CAD build for the part. Positions are in the model's coordinates, mm. A direction names the side the tool comes from. Round coordinates to 2 decimals unless told otherwise and drop trailing zeros. Order: outer loops, then holes, each group sorted by start corner. A loop starts at its lowest first (then second) coordinate and runs counter-clockwise, first axis right, second up. Notation, with made-up numbers: (-38.75, 60) - (-0.75, 60) arc R24 ccw to (-0.75, 77) - close; hole circle Ø10 at (31.5, 79). An arc over 180 degrees is marked (long way). Use one line per item in the form item = value. Start each with the question number.
from build123d import *

# Parameters (mm, degrees)
SKETCH_8_W                = 70
SKETCH_8_H                = 30
EXTRUDE_3_DEPTH           = 60
SKETCH_9_W                = 30
SKETCH_9_H                = 40
SKETCH_9_W_2              = 20
CUT_EXTRUDE_3_DEPTH       = 83.758884896
OTHER_1_OUTLINE_R         = 5.5
OTHER_1_DEPTH             = 5
HOLE_WIZARD_2_D           = 4.5
HOLE_WIZARD_2_DEPTH       = 10
HOLE_WIZARD_2_CBORE_D     = 8
HOLE_WIZARD_2_CBORE_DEPTH = 4.6
BACK_REACH                = 85.4
SKETCH_16_W               = 70
SKETCH_16_H               = 8.975361008
MM_1_D                    = 4
MM_1_DEPTH                = 5
MM_1_TIP                  = 1.201721238
CUT_EXTRUDE_5_DEPTH       = 5
SKETCH_24_W               = 5
SKETCH_24_H               = 21.024638992
SKETCH_24_W_2             = 20
CUT_EXTRUDE_6_DEPTH       = 10
HOLE_WIZARD_3_D           = 6.6
HOLE_WIZARD_3_DEPTH       = 10
HOLE_WIZARD_3_CBORE_D     = 11
HOLE_WIZARD_3_CBORE_DEPTH = 6.8
FILLET_1_R                = 2
SKETCH_29_W               = 10
SKETCH_29_H               = 2
EXTRUDE_5_DEPTH           = 2.329281552
FILLET_3_R                = 2


# Read off the part's stored shape, not the designer's step: 孔1
with BuildPart() as part:
    # 草图8 → 凸台-拉伸3 (new body)
    with BuildSketch(Plane(origin=(0, 0, 0), x_dir=(1, 0, 0), z_dir=(0, 1, 0))):
        with Locations((13.466824006, -16.724598186)):
            Rectangle(SKETCH_8_W, SKETCH_8_H)
    extrude(amount=EXTRUDE_3_DEPTH)

    # 草图9 → 切除-拉伸3 (cut, through all)
    with BuildSketch(Plane.XY.offset(31.724598186)):
        with Locations((-6.533175994, 30)):
            Rectangle(SKETCH_9_W, SKETCH_9_H)
        with Locations((38.466824006, 30)):
            Rectangle(SKETCH_9_W_2, SKETCH_9_H)
    extrude(amount=-CUT_EXTRUDE_3_DEPTH, mode=Mode.SUBTRACT)

    # 孔1 outline → 孔1 (cut)
    with BuildSketch(Plane(origin=(0, 0, 0), x_dir=(1, 0, 0), z_dir=(0, 1, 0))):
        with Locations((-1.490630647, -21.665240746)):
            Circle(OTHER_1_OUTLINE_R)
    extrude(amount=OTHER_1_DEPTH, mode=Mode.SUBTRACT)

    # 打孔尺寸(%根据)内六角圆柱头螺钉的类型2
    with Locations(Plane(origin=(-1.533175994, 10, 21.724598186), x_dir=(1, 0, 0), z_dir=(0, 1, 0))):
        with Locations((0, 0)):
            CounterBoreHole(HOLE_WIZARD_2_D / 2, HOLE_WIZARD_2_CBORE_D / 2, HOLE_WIZARD_2_CBORE_DEPTH, depth=HOLE_WIZARD_2_DEPTH)

    # back: up to this face of the body (flat: up to its plane)
    back_end = Plane(part.part.faces().sort_by_distance((-6.533175994, 50, 16.724598186))[0])
    # 草图16 → back (cut, up to the picked face)
    with BuildSketch(Plane(origin=(0, 0, 0), x_dir=(1, 0, 0), z_dir=(0, 1, 0)), mode=Mode.PRIVATE) as back_sk1:
        with Locations((13.466824006, -6.21227869)):
            Rectangle(SKETCH_16_W, SKETCH_16_H)
    back_tool1 = split(extrude(back_sk1.sketch, amount=BACK_REACH, mode=Mode.PRIVATE), bisect_by=back_end, keep=Keep.BOTH, mode=Mode.PRIVATE)
    add(back_tool1.solids().sort_by(Axis((13.466824, 0, 6.212279), (0, 1, 0)))[0], mode=Mode.SUBTRACT)

    # 大小mm 暗销孔1
    with Locations(Plane(origin=(-1.533175994, 60, 11.724598186), x_dir=(0, 0, 1), z_dir=(0, 1, 0))):
        with Locations((0, 0)):
            Hole(MM_1_D / 2, depth=MM_1_DEPTH)
            with Locations((0, 0, -(MM_1_DEPTH + MM_1_TIP / 2))):  # 118° drill point
                Cone(0, MM_1_D / 2, MM_1_TIP, mode=Mode.SUBTRACT)

    # 草图23 → 切除-拉伸5 (cut)
    with BuildSketch(Plane.XZ.offset(-60)):
        with BuildLine():
            Line((29.466824006, 9.724598186), (27.466824006, 9.724598186))
            ThreePointArc((27.466824006, 9.724598186), (25.466824006, 11.724598186), (27.466824006, 13.724598186))
            Line((27.466824006, 13.724598186), (29.466824006, 13.724598186))
            ThreePointArc((29.466824006, 13.724598186), (31.466824006, 11.724598186), (29.466824006, 9.724598186))
        make_face()
    extrude(amount=CUT_EXTRUDE_5_DEPTH, mode=Mode.SUBTRACT)

    # 草图24 → 切除-拉伸6 (cut)
    with BuildSketch(Plane(origin=(0, 0, 0), x_dir=(1, 0, 0), z_dir=(0, 1, 0))):
        with Locations((-19.033175994, -21.21227869)):
            Rectangle(SKETCH_24_W, SKETCH_24_H)
        with Locations((38.466824006, -21.21227869)):
            Rectangle(SKETCH_24_W_2, SKETCH_24_H)
    extrude(amount=CUT_EXTRUDE_6_DEPTH, mode=Mode.SUBTRACT)

    # 打孔尺寸(%根据)内六角圆柱头螺钉的类型3
    with Locations(Plane(origin=(-11.533175994, 50, 11.724598186), x_dir=(0, 0, -1), z_dir=(0, -1, 0))):
        with Locations((0, 0), (0, 50)):
            CounterBoreHole(HOLE_WIZARD_3_D / 2, HOLE_WIZARD_3_CBORE_D / 2, HOLE_WIZARD_3_CBORE_DEPTH, depth=HOLE_WIZARD_3_DEPTH)

    # 圆角1
    fillet_1_edges = [part.edges().sort_by_distance(p)[0] for p in [
        (-16.533175994, 0, 21.21227869),
        (-16.533175994, 10, 21.21227869),
        (28.466824006, 0, 21.21227869),
        (-21.533175994, 50, 16.724598186),
        (48.466824006, 50, 16.724598186),
        (8.466824006, 50, 21.21227869),
        (28.466824006, 50, 21.21227869),
    ]]
    fillet(fillet_1_edges, radius=FILLET_1_R)

    # 草图29 → 凸台-拉伸5 (add)
    with BuildSketch(Plane(origin=(0, 0, 10.699959194), x_dir=(-1, 0, 0), z_dir=(0, 0, -1))):
        with Locations((0, -1)):
            Rectangle(SKETCH_29_W, SKETCH_29_H)
    extrude(amount=-EXTRUDE_5_DEPTH)

    # 圆角3
    fillet_3_edges = [part.edges().sort_by_distance(p)[0] for p in [
        (-5, -2, 11.86459997),
        (5, -2, 11.86459997),
    ]]
    fillet(fillet_3_edges, radius=FILLET_3_R - 0.0001)  # a hair under: the kernel refuses the full size


solid = part.part
(1) Slice it at A-A (x = 12). Give the cut face in (y, z), and give its area (3 significant figures).
(2) Which spindle directions (+Z, -Z, +X, -X, +Y, -Y) get a long thin tool onto all of the face, cutting with end or side? Do faces 1 (the cylindrical face through (-15.96, 9.4, 21.07)), 2 (the flat face through (28, 58, 9.725)), 3 (the flat face through (6, 50, 17)). Say none if no direction does.
(3) Flat gauge pins, fed straight in: P1, Ø10.5, axis at y = 35, z = 22.5, coming from the -X side; P2, Ø9, axis at x = 40.5, z = 9.5, coming from the -Y side; P3, Ø1, axis at y = 28, z = 16.5, coming from the +X side; P4, Ø1, axis at y = 32, z = 9, coming from the -X side. Where does each tip first touch, or does it go through?
(4) Slice it at B-B (z = 28.5). Give the cut face in (x, y), and give its area (3 significant figures).
(5) Slice it at C-C (x = -13.5). Give the cut face in (y, z).
(6) Mould opens along Y. For faces 4 (the flat face through (13, 30, 31.725)), 5 (the flat face through (0, -2, 12)), 6 (the flat face through (-14, 56.8, 9)) say: pulls with the +Y half, pulls with the -Y half, needs draft (parallel to the pull), parting line crosses it, or undercut.
(7) Slice it at D-D (y = 26). Give the cut face in (x, z), and give its area (3 significant figures).
(8) Wall check: line 1 (Y direction, x = -12, z = 30.75); line 2 (Y direction, x = 31.5, z = 28); line 3 (Z direction, x = 18, y = 41). Give the ranges that are in metal, low to high. Write a range as [from, to].
Results list:
q1.outline = (0, 10.7) - (50, 10.7) - (50, 1.72) - (60, 1.72) - (60, 31.72) - (0, 31.72) - close
q1.area = 1,350 mm²
q2.face_1 = +Z, -Z, -X
q2.face_2 = +Y
q2.face_3 = -Z
q3.P1 = 8.47
q3.P2 = 50
q3.P3 = 28.47
q3.P4 = through
q4.outline = (-21.53, 52) arc R2 ccw to (-19.53, 50) - (6.47, 50) arc R2 cw to (8.47, 48) - (8.47, 10) - (-14.53, 10) arc R2 ccw to (-16.53, 8) - (-16.53, 2) arc R2 ccw to (-14.53, 0) - (26.47, 0) arc R2 ccw to (28.47, 2) - (28.47, 48) arc R2 cw to (30.47, 50) - (46.47, 50) arc R2 ccw to (48.47, 52) - (48.47, 60) - (-21.53, 60) - close
q4.area = 1,950 mm²
q5.outline = (0, 10.7) - (10, 10.7) - (10, 31.72) - (0, 31.72) - close; (50, 1.72) - (60, 1.72) - (60, 9.07) - (56.8, 9.07) - (56.8, 6.59) - (50, 6.59) - close; (50, 16.86) - (56.8, 16.86) - (56.8, 14.37) - (60, 14.37) - (60, 31.72) - (50, 31.72) - close
q6.face_4 = needs draft
q6.face_5 = pulls with the -Y half
q6.face_6 = undercut
q7.outline = (8.47, 10.7) - (28.47, 10.7) - (28.47, 31.72) - (8.47, 31.72) - close
q7.area = 420 mm²
q8.line_1 = [0, 10], [50, 60]
q8.line_2 = [50, 60]
q8.line_3 = [10.7, 31.72]
